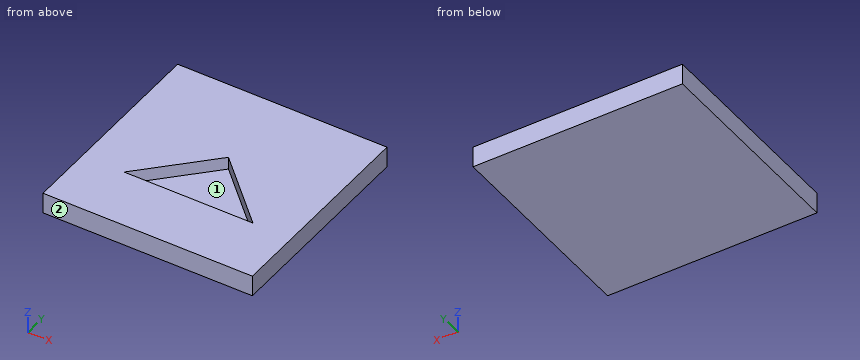
from build123d import *

# Parameters (mm, degrees)
PAD_DEPTH    = 12
SKETCH001_W  = 100
SKETCH001_H  = 100
PAD001_DEPTH = 10


with BuildPart() as body:
    # Sketch → Pad (new body)
    with BuildSketch(Plane.XY):
        Polygon((-30.054117, -20.75305), (31.468237, -20.75305), (0, 10), align=None)
    extrude(amount=PAD_DEPTH)


with BuildPart() as body_1:
    # Body placement: moved
    add(body.part.moved(Location((0, 0, -6))))


with BuildPart() as model_cut:
    # Sketch001 → Pad001 (new body)
    with BuildSketch(Plane.XY):
        Rectangle(SKETCH001_W, SKETCH001_H)
    extrude(amount=PAD001_DEPTH)


with BuildPart() as model_cut_1:
    # Body001 placement: moved
    add(model_cut.part.moved(Location((0, 0, -10))))

    # Cut: cut Body
    add(body_1.part, mode=Mode.SUBTRACT)


solid = model_cut_1.part
Can you work these out from the model? Positions are in its coordinate system, mm. Face numbers are marked on the shaded views. A direction names the side the tool comes from. Give positions to 0.01 mm unless a question says otherwise; leave off trailing zeros. Write each loop counter-clockwise with the first axis right and the second up, starting at its lowest first coordinate (ties: lowest second). Pieces come first, ordered by that corner, then holes. Notation, with made-up numbers: M -22.5,89 L 15.5,89 A24 cw 15.5,116 Z; hole C -20.75,72 d1. An arc over 180 degrees is marked long. Answer in a Markdown table with one row per item. Add a question column.
Item 1: For pin 1 Ø9 at (x, y) = (1.5, -7) entering from +Z, with a flat end and sliding along its axis, tell me the tip position at first contact or that it passes through.
Item 2: Imagine slicing it at B-B, the plane y = -3. Write out the boundary of the cut face in (x, z), plus the area to 3 significant figures.
Item 3: Please list where these lines run through material, in increasing order: L1, parallel to Y at x = -4, z = -0.75; L2, parallel to Y at x = 7, z = -2.75; L3, parallel to X at y = -11.5, z = -2.
Item 4: On a 3-axis mill with a long thin cutter (end or side, diameter ignored), from which of +Z, -Z, +X, -X, +Y, -Y can I reach the whole of each face in a straight line? I mean the marked faces 1 and 2. Say none if no direction works.
Item 5: Imagine slicing it at C-C, the plane x = 25. Write out the boundary of the cut face in (y, z), plus the area to 3 significant figures.
Item 6: Imagine slicing it at A-A, the plane z = -4.5. Write out the boundary of the cut face in (x, y).
Evaluation:
| question | item | result |
|---|---|---|
| 1 | pin 1 | stops at z = -6 |
| 2 | outline | M -50,-10 L 50,-10 L 50,0 L 13.3,0 L 13.3,-6 L -12.7,-6 L -12.7,0 L -50,0 Z |
| 2 | area | 844 mm² |
| 3 | L1 | y = -50 to -20.75, 5.91 to 50 |
| 3 | L2 | y = -50 to -20.75, 3.16 to 50 |
| 3 | L3 | x = -50 to -21.01, 22 to 50 |
| 4 | face 1 | +Z |
| 4 | face 2 | +Z, -Z, +X, -X, -Y |
| 5 | outline | M -50,-10 L 50,-10 L 50,0 L -14.43,0 L -14.43,-6 L -20.75,-6 L -20.75,0 L -50,0 Z |
| 5 | area | 962 mm² |
| 6 | outline | M -50,-50 L 50,-50 L 50,50 L -50,50 Z; hole M -30.05,-20.75 L 31.47,-20.75 L 0,10 Z |
